Model file for the job. Use its own axes, mm. A direction names the side the tool comes from. Coordinates: 2 decimals unless noted, no trailing zeros. Write each loop counter-clockwise with the first axis right and the second up, starting at its lowest first coordinate (ties: lowest second). Pieces come first, ordered by that corner, then holes. Notation, with made-up numbers: (-27.75, -15) -> (-20.75, -15) arc R17 cw to (-20.75, 15) -> close; hole circle Ø11 at (54.5, 47). An arc over 180 degrees is marked (long way). Answer as a JSON object with one key per item and string values. Group by question number.
from build123d import *

# Parameters (mm, degrees)
SKETCH1_R           = 4
BOSS_EXTRUDE1_DEPTH = 15
SKETCH2_R           = 3
BOSS_EXTRUDE2_DEPTH = 59.52
SKETCH3_R           = 2.425
SKETCH3_R_2         = 1.02
CUT_EXTRUDE1_DEPTH  = 4
SKETCH4_R           = 3
BOSS_EXTRUDE3_DEPTH = 4
SKETCH5_R           = 1.5
CUT_EXTRUDE2_DEPTH  = 50


with BuildPart() as part:
    # Sketch1 → Boss-Extrude1 (new body)
    with BuildSketch(Plane(origin=(0, 0, 0), x_dir=(1, 0, 0), z_dir=(0, 1, 0))):
        Circle(SKETCH1_R)
    extrude(amount=BOSS_EXTRUDE1_DEPTH)

    # Sketch2 → Boss-Extrude2 (add)
    with BuildSketch(Plane(origin=(0, 15, 0), x_dir=(1, 0, 0), z_dir=(0, 1, 0))):
        Circle(SKETCH2_R)
    extrude(amount=BOSS_EXTRUDE2_DEPTH)

    # Sketch3 → Cut-Extrude1 (cut)
    with BuildSketch(Plane.XZ):
        Circle(SKETCH3_R)
        Circle(SKETCH3_R_2, mode=Mode.SUBTRACT)
    extrude(amount=-CUT_EXTRUDE1_DEPTH, mode=Mode.SUBTRACT)

    # Sketch4 → Boss-Extrude3 (add)
    with BuildSketch(Plane(origin=(0, 74.52, 0), x_dir=(1, 0, 0), z_dir=(0, 1, 0))):
        Circle(SKETCH4_R)
    extrude(amount=BOSS_EXTRUDE3_DEPTH)

    # Sketch5 → Cut-Extrude2 (cut)
    with BuildSketch(Plane(origin=(0, 78.52, 0), x_dir=(1, 0, 0), z_dir=(0, 1, 0))):
        Circle(SKETCH5_R)
    extrude(amount=-CUT_EXTRUDE2_DEPTH, mode=Mode.SUBTRACT)


solid = part.part
(1) Cut at D-D on y = 22.5. List the corners of the cut face in (x, z), plus the area to 3 significant figures.
(2) Cut at B-B on z = 0. List the corners of the cut face in (x, y) (3 decimals).
(3) Pin check, flat tips, straight feed: pin 1 (1 mm diameter, centred on y = 49.5, z = -3, fed in from +X); pin 2 (2 mm diameter, centred on x = -2, y = 56, fed in from -Z); pin 3 (1 mm diameter, centred on y = 35, z = 0.5, fed in from +X). Stop position of each tip, or through.
(4) 3-axis set-ups, long thin cutter, end or side, ignore diameter. For faces 1 (the face through (0, 0, 0)), 2 (the face through (0, 28.52, 0)), 3 (the face through (-0.81, 1.97, -0.62)): which of +Z, -Z, +X, -X, +Y, -Y reach the whole face in a straight line?
(5) Wall check: probe 1 along Z at (x, y) = (0, 1.6) (3 decimals); probe 2 along X at (y, z) = (66, 0). Give the ranges that are in metal, low to high.
(6) Cut at A-A on x = 0. List the corners of the cut face in (y, z) (3 decimals).
(7) Pull direction X, two halves, no side cores. Call faces 4 (the face through (-1.5, 53.87, -0.07)), 5 (the face through (1, 15, -3)), 6 (the face through (-0.867, 7.395, 3.905)): released by +X, released by -X, zero draft, split by the parting line, or undercut.
(8) Cut at C-C on y = 56. List the corners of the cut face in (x, z), plus the area to 3 significant figures.
Results found:
{
 "1": {"outline": "circle Ø6 at (0, 0)", "area": "28.3 mm²"},
 "2": {"outline": "(-4, 0) -> (-2.425, 0) -> (-2.425, 4) -> (-1.02, 4) -> (-1.02, 0) -> (1.02, 0) -> (1.02, 4) -> (2.425, 4) -> (2.425, 0) -> (4, 0) -> (4, 15) -> (3, 15) -> (3, 78.52) -> (1.5, 78.52) -> (1.5, 28.52) -> (-1.5, 28.52) -> (-1.5, 78.52) -> (-3, 78.52) -> (-3, 15) -> (-4, 15) -> close"},
 "3": {"pin 1": "stops at x = 1.66", "pin 2": "stops at z = -2.83", "pin 3": "stops at x = 3"},
 "4": {"face 1": "+Z, -Z, +X, -X, -Y", "face 2": "+Y", "face 3": "-Y"},
 "5": {"probe 1": "z = -4 to -2.425, -1.02 to 1.02, 2.425 to 4", "probe 2": "x = -3 to -1.5, 1.5 to 3"},
 "6": {"outline": "(0, -4) -> (15, -4) -> (15, -3) -> (78.52, -3) -> (78.52, -1.5) -> (28.52, -1.5) -> (28.52, 1.5) -> (78.52, 1.5) -> (78.52, 3) -> (15, 3) -> (15, 4) -> (0, 4) -> (0, 2.425) -> (4, 2.425) -> (4, 1.02) -> (0, 1.02) -> (0, -1.02) -> (4, -1.02) -> (4, -2.425) -> (0, -2.425) -> close"},
 "7": {"face 4": "undercut", "face 5": "zero draft", "face 6": "split by the parting line"},
 "8": {"outline": "circle Ø6 at (0, 0); hole circle Ø3 at (0, 0)", "area": "21.2 mm²"}
}
